Can you work these out from the model? Positions are in its coordinate system, mm. A direction names the side the tool comes from. Coordinates: 2 decimals unless noted, no trailing zeros. Order: outer loops, then holes, each group sorted by start corner. A loop starts at its lowest first (then second) coordinate and runs counter-clockwise, first axis right, second up. Notation, with made-up numbers: (-7, 28.25) -> (48, 28.25) arc R22 ccw to (48, 65.25) -> close; hole circle Ø1 at (40.25, 37). An arc over 180 degrees is marked (long way). Use a Markdown table: item, result. Add a question column.
1. For faces 4 (the flat face through (2, 0, 0)), 5 (the cylindrical face through (-19.93, 5.54, 42.06)), 6 (the flat face through (-25, 5, 45)), which set-ups out of +Z, -Z, +X, -X, +Y, -Y let a thin tool reach every point of the face, with its end or its side?
2. Suppose I cut it at B-B, the plane z = 44.5. List the corners of the cut face in (x, y) for me.
3. We'd pull the mould along Y, two halves only. Please class faces 1 (the cylindrical face through (-34.171, 1.881, 28.827)), 2 (the flat face through (-25, -5, 45)), 3 (the cylindrical face through (-19.93, -4.46, 42.06)): pulls with the +Y half, pulls with the -Y half, needs draft (parallel to the pull), parting line crosses it, or undercut.
4. Suppose I cut it at C-C, the plane z = 14.5. List the corners of the cut face in (x, y) for me.
5. Suppose I cut it at A-A, the plane y = 0. List the corners of the cut face in (x, z) for me.
6. For pin 1 Ø5 at (x, y) = (-46, -2) entering from +Z; pin 2 Ø15.5 at (y, z) = (-1.5, 41.5) entering from -X; pin 3 Ø3 at (x, y) = (-13.5, -2.5) entering from -Z, each with a flat end and sliding along its axis, tell me the tip position at first contact or that it passes through.
7. If I drill on line 1 along X through (y, z) = (-7.5, 36.5); line 2 along Z through (x, y) = (-13, 2.25); line 3 along Z through (x, y) = (-20, -4.75), over which ranges is the centre line in solid material (lowest first)? Write a range as from..to.
8. Suppose I cut it at D-D, the plane y = 10.25. List the corners of the cut face in (x, z) for me.
```python
from build123d import *

# Parameters (mm, degrees)
F0_W     = 30
F0_H     = 30
F1_DEPTH = 48.5
F2_W     = 4
F2_H     = 30
F3_DEPTH = 29
F4_R     = 14.45
F5_DEPTH = 47
F6_R     = 2.5
F7_DEPTH = 10


with BuildPart() as f1:
    # F0 (on Top) → F1 (new body)
    with BuildSketch(Plane.XY):
        Rectangle(F0_W, F0_H)
    extrude(amount=F1_DEPTH)

    # F2 (on face) → F3 (cut)
    with BuildSketch(Plane(origin=(0, 0, 0), x_dir=(1, 0, 0), z_dir=(0, 0, -1))):
        with Locations((-13, 0)):
            Rectangle(F2_W, F2_H)
    extrude(amount=-F3_DEPTH, mode=Mode.SUBTRACT)

    # F4 (on face) → F5 (join)
    with BuildSketch(Plane(origin=(-11, 0, 0), x_dir=(0, -1, 0), z_dir=(-1, 0, 0))):
        with Locations((0, 14.5)):
            Circle(F4_R)
    extrude(amount=F5_DEPTH)

    # F6 (on face) → F7 (join)
    with BuildSketch(Plane(origin=(-15, 0, 0), x_dir=(0, -1, 0), z_dir=(-1, 0, 0))):
        with Locations((5, 44.5)):
            Circle(F6_R)
        with Locations((-5, 44.5)):
            Circle(F6_R)
    extrude(amount=F7_DEPTH)


solid = f1.part
```
Worked out:
| question | item | result |
|---|---|---|
| 1 | face 4 | -Z, +X, -X, +Y, -Y |
| 1 | face 5 | -X |
| 1 | face 6 | +Z, -X, +Y, -Y |
| 2 | outline | (-25, -7.5) -> (-15, -7.5) -> (-15, -15) -> (15, -15) -> (15, 15) -> (-15, 15) -> (-15, 7.5) -> (-25, 7.5) -> (-25, 2.5) -> (-15, 2.5) -> (-15, -2.5) -> (-25, -2.5) -> close |
| 3 | face 1 | parting line crosses it |
| 3 | face 2 | needs draft |
| 3 | face 3 | undercut |
| 4 | outline | (-58, -14.45) -> (-11, -14.45) -> (-11, -15) -> (15, -15) -> (15, 15) -> (-11, 15) -> (-11, 14.45) -> (-58, 14.45) -> close |
| 5 | outline | (-58, 0.05) -> (-11, 0.05) -> (-11, 0) -> (15, 0) -> (15, 48.5) -> (-15, 48.5) -> (-15, 29) -> (-11, 29) -> (-11, 28.95) -> (-58, 28.95) -> close |
| 6 | pin 1 | stops at z = 28.95 |
| 6 | pin 2 | stops at x = -25 |
| 6 | pin 3 | stops at z = 0.08 |
| 7 | line 1 | x = -15..15 |
| 7 | line 2 | z = 0.23..28.77, 29..48.5 |
| 7 | line 3 | z = 0.85..28.15, 42.01..46.99 |
| 8 | outline | (-58, 4.31) -> (-11, 4.31) -> (-11, 0) -> (15, 0) -> (15, 48.5) -> (-15, 48.5) -> (-15, 29) -> (-11, 29) -> (-11, 24.69) -> (-58, 24.69) -> close |
